Input: part model. Units: mm. Frame: model coordinates. A direction names the side the tool comes from. Give positions to 0.01 mm unless a question says otherwise; leave off trailing zeros. Loops run counter-clockwise (first coordinate to the right, second up) from the corner with the lowest first, then second, coordinate; pieces in that order, holes last.
from build123d import *

# Parameters (mm, degrees)
SKETCH_1_W          = 23
SKETCH_1_H          = 23
SKETCH_1_W_2        = 13
SKETCH_1_H_2        = 13
EXTRUDE_1_DEPTH     = 53.9
SKETCH_2_R          = 1.65
CUT_EXTRUDE_1_DEPTH = 34
SKETCH_4_W          = 23
SKETCH_4_H          = 23
SKETCH_4_R          = 3
EXTRUDE_2_DEPTH     = 14.6
SKETCH_5_W          = 23
SKETCH_5_H          = 23
SKETCH_5_W_2        = 13
SKETCH_5_H_2        = 13
EXTRUDE_1_2_DEPTH   = 10
SKETCH_6_R          = 1.65
CUT_EXTRUDE_2_DEPTH = 39
SKETCH_7_W          = 13
SKETCH_7_H          = 13
CUT_EXTRUDE_3_DEPTH = 24.6
CHAMFER_1_SIZE      = 3
SKETCH_8_W          = 47.6
SKETCH_8_H          = 53.9
CUT_EXTRUDE_4_DEPTH = 11.5
EXTRUDE_3_DEPTH     = 6.5
FILLET_1_R          = 10
FILLET_2_R          = 10
SKETCH_10_R         = 1.65
CUT_EXTRUDE_5_DEPTH = 28.5
CHAMFER_3_SIZE      = 3
CHAMFER_4_SIZE      = 3
CHAMFER_5_SIZE      = 3


with BuildPart() as part:
    # 草图1 → Extrude 1 (new body)
    with BuildSketch(Plane.XY):
        with Locations((6.5, 6.5)):
            Rectangle(SKETCH_1_W, SKETCH_1_H)
        with Locations((6.5, 6.5)):
            Rectangle(SKETCH_1_W_2, SKETCH_1_H_2, mode=Mode.SUBTRACT)
    extrude(amount=EXTRUDE_1_DEPTH)

    # 草图2 → 切除-拉伸1 (cut)
    with BuildSketch(Plane.XZ.offset(5)):
        with Locations(Location((6.5, 43.9, 0), (0, 0, 270))):
            Circle(SKETCH_2_R)
    extrude(amount=-CUT_EXTRUDE_1_DEPTH, mode=Mode.SUBTRACT)

    # 草图4 → 凸台-拉伸2 (add)
    with BuildSketch(Plane(origin=(18, 0, 0), x_dir=(0, 0, -1), z_dir=(1, 0, 0))):
        with Locations((-11.5, 6.5)):
            Rectangle(SKETCH_4_W, SKETCH_4_H)
        with Locations(Location((-11.5, 6.5, 0), (0, 0, 90))):
            Circle(SKETCH_4_R, mode=Mode.SUBTRACT)
    extrude(amount=EXTRUDE_2_DEPTH)

    # 草图5 → Extrude 1 2 (add)
    with BuildSketch(Plane(origin=(32.6, 0, 0), x_dir=(0, 0, -1), z_dir=(1, 0, 0))):
        with Locations((-11.5, 6.5)):
            Rectangle(SKETCH_5_W, SKETCH_5_H)
        with Locations((-11.5, 6.5)):
            Rectangle(SKETCH_5_W_2, SKETCH_5_H_2, mode=Mode.SUBTRACT)
    extrude(amount=EXTRUDE_1_2_DEPTH)

    # 草图6 → 切除-拉伸2 (cut)
    with BuildSketch(Plane(origin=(0, 18, 0), x_dir=(1, 0, 0), z_dir=(0, 1, 0))):
        with Locations(Location((32.6, -11.5, 0), (0, 0, 270))):
            Circle(SKETCH_6_R)
    extrude(amount=-CUT_EXTRUDE_2_DEPTH, mode=Mode.SUBTRACT)

    # 草图7 → 切除-拉伸3 (cut)
    with BuildSketch(Plane(origin=(32.6, 0, 0), x_dir=(0, 0, -1), z_dir=(1, 0, 0))):
        with Locations((-11.5, 6.5)):
            Rectangle(SKETCH_7_W, SKETCH_7_H)
    extrude(amount=-CUT_EXTRUDE_3_DEPTH, mode=Mode.SUBTRACT)

    # 倒角1
    chamfer_1_edges = [part.edges().sort_by_distance(p)[0] for p in [
        (13, 6.5, 18),
    ]]
    chamfer(chamfer_1_edges, length=CHAMFER_1_SIZE)

    # 草图8 → 切除-拉伸4 (cut)
    with BuildSketch(Plane.XZ.offset(5)):
        with Locations((18.8, 26.95)):
            Rectangle(SKETCH_8_W, SKETCH_8_H)
    extrude(amount=-CUT_EXTRUDE_4_DEPTH, mode=Mode.SUBTRACT)

    # 草图9 → 凸台-拉伸3 (add)
    with BuildSketch(Plane.XZ.offset(-13)):
        Polygon((13, 5), (0, 18), (0, 0), (13, 0), align=None)
    extrude(amount=EXTRUDE_3_DEPTH)

    # 圆角1
    fillet_1_edges = [part.edges().sort_by_distance(p)[0] for p in [
        (-5, 12.25, 0),
    ]]
    fillet(fillet_1_edges, radius=FILLET_1_R)

    # 圆角2
    fillet_2_edges = [part.edges().sort_by_distance(p)[0] for p in [
        (18, 12.25, 23),
    ]]
    fillet(fillet_2_edges, radius=FILLET_2_R)

    # 草图10 → 切除-拉伸5 (cut)
    with BuildSketch(Plane.XZ.offset(-6.5)):
        with Locations(Location((2, 7, 0), (0, 0, 270))):
            Circle(SKETCH_10_R)
        with Locations(Location((18, 23, 0), (0, 0, 270))):
            Circle(SKETCH_10_R)
    extrude(amount=-CUT_EXTRUDE_5_DEPTH, mode=Mode.SUBTRACT)

    # 倒角3
    # the kernel refuses this chamfer: 3 mm, written as the material it takes off along each edge
    with BuildSketch(Plane(origin=(5, 18, 10), x_dir=(0, 0, -1), z_dir=(1, 0, 0))) as chamfer_3_piece_1:
        Polygon((10 - CHAMFER_3_SIZE, 0), (10, -CHAMFER_3_SIZE), (10, 0), align=None)
    revolve(axis=Axis((5, 18, 10), (0, 1, 0)), revolution_arc=90, mode=Mode.SUBTRACT)
    with BuildSketch(Plane(origin=(28, 18, 33), x_dir=(-1, 0, 0), z_dir=(0, 0, 1))) as chamfer_3_piece_2:
        Polygon((10 + CHAMFER_3_SIZE, 0), (10, CHAMFER_3_SIZE), (10, 0), align=None)
    revolve(axis=Axis((28, 18, 33), (0, -1, 0)), revolution_arc=90, mode=Mode.SUBTRACT)
    with BuildSketch(Plane(origin=(28, 18, 23), x_dir=(0, 0.027495876610586768, -0.9996219169112968), z_dir=(1, 0, 0))) as chamfer_3_piece_3:
        Polygon((CHAMFER_3_SIZE * 0.999621916911, -CHAMFER_3_SIZE * 0.0274958766106), (-CHAMFER_3_SIZE * 0.0274958766106, -CHAMFER_3_SIZE * 0.999621916911), (0, 0), align=None)
    extrude(amount=22.315048964, mode=Mode.SUBTRACT)
    with BuildSketch(Plane(origin=(50.315048964, 18, 0), x_dir=(0, 0.027495876610586778, 0.9996219169112968), z_dir=(-1, 0, 0))) as chamfer_3_piece_4:
        Polygon((CHAMFER_3_SIZE * 0.999621916911, -CHAMFER_3_SIZE * 0.0274958766106), (-CHAMFER_3_SIZE * 0.0274958766106, -CHAMFER_3_SIZE * 0.999621916911), (0, 0), align=None)
    extrude(amount=45.315048964, mode=Mode.SUBTRACT)
    with BuildSketch(Plane(origin=(-5, 18, 10), x_dir=(0.9996219169112968, 0.027495876610586778, 0), z_dir=(0, 0, 1))) as chamfer_3_piece_5:
        Polygon((CHAMFER_3_SIZE * 0.999621916911, -CHAMFER_3_SIZE * 0.0274958766106), (-CHAMFER_3_SIZE * 0.0274958766106, -CHAMFER_3_SIZE * 0.999621916911), (0, 0), align=None)
    extrude(amount=51.615048964, mode=Mode.SUBTRACT)
    with BuildSketch(Plane(origin=(18, 18, 33), x_dir=(-0.9996219169112968, 0.02749587661058678, 0), z_dir=(0, 0, 1))) as chamfer_3_piece_6:
        Polygon((CHAMFER_3_SIZE * 0.999621916911, CHAMFER_3_SIZE * 0.0274958766106), (-CHAMFER_3_SIZE * 0.0274958766106, CHAMFER_3_SIZE * 0.999621916911), (0, 0), align=None)
    extrude(amount=28.615048964, mode=Mode.SUBTRACT)

    # 倒角4
    chamfer_4_edges = [part.edges().sort_by_distance(p)[0] for p in [
        (42.6, 18, 11.5),
        (6.5, 18, 53.9),
    ]]
    chamfer(chamfer_4_edges, length=CHAMFER_4_SIZE)

    # 倒角5
    chamfer_5_edges = [part.edges().sort_by_distance(p)[0] for p in [
        (42.6, 10.75, 0),
        (18, 10.75, 53.9),
        (-5, 10.75, 53.9),
        (42.6, 10.75, 23),
    ]]
    chamfer(chamfer_5_edges, length=CHAMFER_5_SIZE)


solid = part.part
(1) Mould query, pull axis X, two halves, no side actions, for faces 1 (the flat face through (22, 11, 0)), 2 (the flat face through (16, 17, 43)), 3 (the flat face through (0, 10, 36)). Classes: +X half, -X half, draft (parallel to the pull), parting line (faces both ways), or undercut.
Values follow:
face 1: draft
face 2: +X half
face 3: undercut
(2) Pin query (flat end, axial travel): pin 1 Ø1.5 at (y, z) = (15, 32.5) entering from +X; pin 2 Ø2 at (y, z) = (9, 38.5) entering from +X; pin 3 Ø3 at (x, y) = (20.5, 11) entering from +Z. Return the tip coordinate at first contact, or that it passes through.
Values follow:
pin 1: stops at x = 18.08
pin 2: stops at x = 18
pin 3: stops at z = 28.64
(3) Cut plane D-D (z = 34). Return the cut outline in (x, y).
Values follow:
outline: (-5, 6.5) - (0, 6.5) - (0, 13) - (13, 13) - (13, 6.5) - (18, 6.5) - (18, 15) - (15, 18) - (-2, 18) - (-5, 15) - close
(4) Reachability of faces 4 (the flat face through (28, 10, 5)), 5 (the flat face through (12, 13, 24)), 6 (the flat face through (13, 10, 37)) from +Z, -Z, +X, -X, +Y, -Y: full face, straight path, thin tool, end or side. Return the list, or none.
Values follow:
face 4: +X, -Y
face 5: -Y
face 6: +Z, -Y
(5) Cut plane B-B (z = 11.5). Return the cut outline in (x, y).
Values follow:
outline: (-5, 6.5) - (6.5, 6.5) - (6.5, 13) - (30.95, 13) - (30.95, 18) - (-2, 18) - (-5, 15) - close; (34.25, 13) - (42.6, 13) - (42.6, 15) - (39.6, 18) - (34.25, 18) - close
(6) Cut plane A-A (y = 10). Return the cut outline in (x, z), and give its area (3 significant figures).
Values follow:
outline: (-5, 10) arc R10 ccw to (5, 0) - (39.6, 0) - (42.6, 3) - (42.6, 5) - (13, 5) - (0, 18) - (0, 53.9) - (-2, 53.9) - (-5, 50.9) - close; (13, 21) - (16, 18) - (42.6, 18) - (42.6, 20) - (39.6, 23) - (28, 23) arc R10 cw to (18, 33) - (18, 50.9) - (15, 53.9) - (13, 53.9) - close; hole circle Ø3.3 at (2, 7); hole circle Ø3.3 at (18, 23)
area: 830 mm2
(7) Ray query, probe 1 along X at (y, z) = (12, 47); probe 2 along X at (y, z) = (14.25, 50); probe 3 along Y at (x, z) = (36, 9.5). Return the intervals inside material, ascending.
Values follow:
probe 1: x = -5 to 0, 13 to 18
probe 2: x = -5 to 18
probe 3: y = 13 to 18
(8) Cut plane C-C (x = 6.5). Return the cut outline in (y, z), and give its area (3 significant figures).
Values follow:
outline: (6.5, 0) - (15, 0) - (18, 3) - (18, 42.25) - (13, 42.25) - (13, 11.5) - (6.5, 11.5) - close; (13, 45.55) - (18, 45.55) - (18, 50.9) - (15, 53.9) - (13, 53.9) - close
area: 319 mm2
